The drawing under review shows one solid part. Ordinate dimensions are in mm from its lowest x, y, z. A direction names the side the tool comes from. Coordinates: 2 decimals unless noted, no trailing zeros. Write each loop counter-clockwise with the first axis right and the second up, starting at its lowest first coordinate (ties: lowest second). Pieces come first, ordered by that corner, then holes.
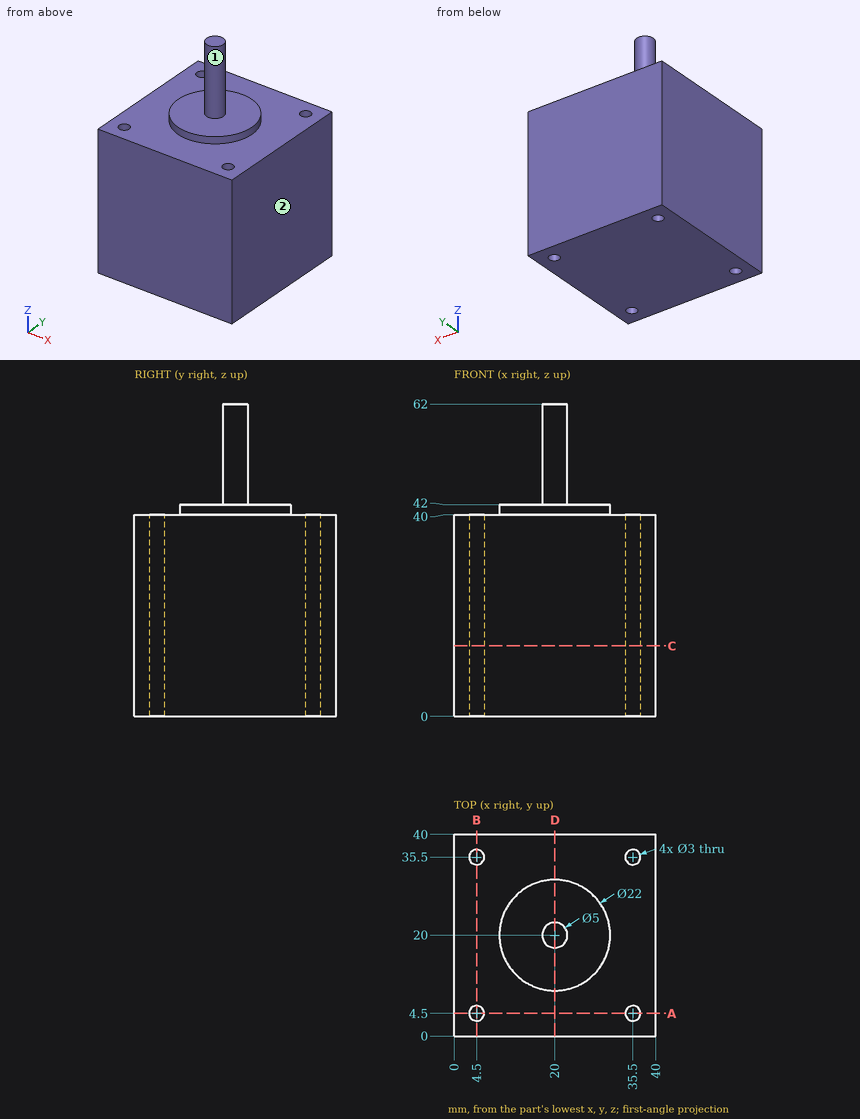
Q1. Add section D-D (x = 20). State the section outline as (y, z) points.
Ans:
outline: (0, 0) - (40, 0) - (40, 40) - (31, 40) - (31, 42) - (22.5, 42) - (22.5, 62) - (17.5, 62) - (17.5, 42) - (9, 42) - (9, 40) - (0, 40) - close
Q2. Tool access review of the marked faces 1 and 2: name each direction out of +Z, -Z, +X, -X, +Y, -Y from which nothing blocks a thin tool from reaching the whole face with its end or side.
Ans:
face 1: +Z
face 2: +Z, -Z, +X, +Y, -Y
Q3. Add section A-A (y = 4.5). State the section outline as (x, z) points, then the cut area to 3 significant figures.
Ans:
outline: (0, 0) - (3, 0) - (3, 40) - (0, 40) - close; (6, 0) - (34, 0) - (34, 40) - (6, 40) - close; (37, 0) - (40, 0) - (40, 40) - (37, 40) - close
area: 1,360 mm2
Q4. Clearance check with flat-ended pins moving along their axes: pin 1 Ø1.5 at (x, y) = (35, 8) entering from +Z; pin 2 Ø3 at (x, z) = (16, 42) entering from -Y. State where each tip first meets the part, or that it passes through.
Ans:
pin 1: stops at z = 40
pin 2: stops at y = 9.29
Q5. Add section C-C (z = 14). State the section outline as (x, y) points.
Ans:
outline: (0, 0) - (40, 0) - (40, 40) - (0, 40) - close; hole circle Ø3 at (4.5, 4.5); hole circle Ø3 at (4.5, 35.5); hole circle Ø3 at (35.5, 4.5); hole circle Ø3 at (35.5, 35.5)
Q6. For probe 1 along Y at (x, z) = (35.5, 21); probe 2 along Y at (x, z) = (4, 22), list the stretches that pass through material, from the lowest coordinate up.
Ans:
probe 1: y = 0 to 3, 6 to 34, 37 to 40
probe 2: y = 0 to 3.09, 5.91 to 34.09, 36.91 to 40
